Build history of the part. All positions in model axes, mm. A direction names the side the tool comes from. Give positions to 0.01 mm unless a question says otherwise; leave off trailing zeros. Loops run counter-clockwise (first coordinate to the right, second up) from the corner with the lowest first, then second, coordinate; pieces in that order, holes last. Notation, with made-up numbers: M 8,83.5 L 22,83.5 A24 ccw 22,100.5 Z; hole C 80.25,33 d2. An arc over 180 degrees is marked long. Put each result on its own line as item: value.
```python
from build123d import *

# Parameters (mm, degrees)
SKETCH_1_W               = 40
SKETCH_1_H               = 40
EXTRUDE_1_DEPTH          = 12.7
CUT_EXTRUDE_2_DEPTH      = 0.7
CUT_EXTRUDE_2_DEPTH_BACK = 1.5
SKETCH_8_W               = 36.4
SKETCH_8_H               = 28.4
CUT_EXTRUDE_4_DEPTH      = 12.7
SKETCH_10_R              = 0.5
SKETCH_10_R_2            = 1.5
SKETCH_10_W              = 3
SKETCH_10_H              = 13
EXTRUDE_2_DEPTH          = 2.2
CUT_EXTRUDE_START        = -12.7
SKETCH_13_R              = 1.35
CUT_EXTRUDE_6_DEPTH      = 12.7
FILLET_1_R               = 1
SKETCH_14_W              = 8.31999735
SKETCH_14_H              = 2.64999918
CUT_EXTRUDE_8_DEPTH      = 5.8
SKETCH_15_W              = 12.8999835
SKETCH_15_H              = 7.3
CUT_EXTRUDE_9_DEPTH      = 5.8
SKETCH_16_W              = 1.085536683
SKETCH_16_H              = 5.100270408
CUT_EXTRUDE_10_DEPTH     = 1.8
SKETCH_17_W              = 8.31999735
SKETCH_17_H              = 2.65925193
CUT_EXTRUDE_11_DEPTH     = 5.8
SKETCH_23_W              = 6.0022214
SKETCH_23_H              = 5.598076211
SKETCH_23_H_2            = 5.598076212
CUT_EXTRUDE_12_DEPTH     = 4
SKETCH_24_W              = 11
SKETCH_24_H              = 14
CUT_EXTRUDE_14_DEPTH     = 1.4


with BuildPart() as part:
    # 草图1 → 凸台-拉伸1 (new body)
    with BuildSketch(Plane(origin=(0, 0, -12.4), x_dir=(-1, 0, 0), z_dir=(0, 0, -1))):
        with Locations((-18.22949197, 11.132690632)):
            Rectangle(SKETCH_1_W, SKETCH_1_H)
    extrude(amount=-EXTRUDE_1_DEPTH)

    # 草图2 → 切除-拉伸2 (cut, two sides: drawn at the far end of the back side and taken through both)
    with BuildSketch(Plane.XY.offset(-8).offset(-CUT_EXTRUDE_2_DEPTH_BACK)):
        Polygon((-2.01828663, -8.469233156), (2.73171337, -8.469233156), (4.23171337, -5.871156945), (2.72949197, -3.269233156), (-2.01828663, -3.269233156), align=None)
        Polygon((-2.01828663, 25.534614421), (-2.01828663, 30.734614421), (2.73171337, 30.734614421), (4.23171337, 28.13653821), (2.72949197, 25.534614421), align=None)
        Polygon((38.47727057, 30.734614421), (33.72727057, 30.734614421), (32.22727057, 28.13653821), (33.72949197, 25.534614421), (38.47727057, 25.534614421), align=None)
        Polygon((38.47727057, -3.269233156), (38.47727057, -8.469233156), (33.72727057, -8.469233156), (32.22727057, -5.871156945), (33.72949197, -3.269233156), align=None)
    extrude(amount=CUT_EXTRUDE_2_DEPTH + CUT_EXTRUDE_2_DEPTH_BACK, mode=Mode.SUBTRACT)

    # 草图8 → 切除-拉伸4 (cut)
    with BuildSketch(Plane(origin=(0, 0, -12.4), x_dir=(-1, 0, 0), z_dir=(0, 0, -1))):
        with Locations((-18.22949197, 11.132690632)):
            Rectangle(SKETCH_8_W, SKETCH_8_H)
    extrude(amount=-CUT_EXTRUDE_4_DEPTH, mode=Mode.SUBTRACT)

    # 草图13 → 切除-拉伸6 (cut)
    with BuildSketch(Plane(origin=(0, 0, -12.4), x_dir=(-1, 0, 0), z_dir=(0, 0, -1)).offset(CUT_EXTRUDE_START)):
        with Locations((-35.22949197, -5.867309368)):
            Circle(SKETCH_13_R)
        with Locations(Location((-1.22949197, -5.867309368, 0), (0, 0, 180))):
            Circle(SKETCH_13_R)
        with Locations((-1.22949197, 28.132690632)):
            Circle(SKETCH_13_R)
        with Locations(Location((-35.22949197, 28.132690632, 0), (0, 0, 180))):
            Circle(SKETCH_13_R)
    extrude(amount=CUT_EXTRUDE_6_DEPTH, mode=Mode.SUBTRACT)

    # 圆角1
    fillet_1_edges = [part.edges().sort_by_distance(p)[0] for p in [
        (0.02949197, 25.332690632, -6.05),
        (0.02949197, -3.067309368, -6.05),
        (36.42949197, -3.067309368, -6.05),
        (36.42949197, 25.332690632, -6.05),
    ]]
    fillet(fillet_1_edges, radius=FILLET_1_R)

    # 草图14 → 切除-拉伸8 (cut)
    with BuildSketch(Plane.XZ.offset(8.867309368)):
        with Locations((8.169941285, -11.07500041)):
            Rectangle(SKETCH_14_W, SKETCH_14_H)
    extrude(amount=-CUT_EXTRUDE_8_DEPTH, mode=Mode.SUBTRACT)

    # 草图15 → 切除-拉伸9 (cut)
    with BuildSketch(Plane.XZ.offset(8.867309368)):
        with Locations((23.79587104, -8.75)):
            Rectangle(SKETCH_15_W, SKETCH_15_H)
    extrude(amount=-CUT_EXTRUDE_9_DEPTH, mode=Mode.SUBTRACT)

    # 草图16 → 切除-拉伸10 (cut)
    with BuildSketch(Plane(origin=(38.22949197, 0, 0), x_dir=(0, 0, -1), z_dir=(1, 0, 0))):
        with Locations((11.857231659, 0.566559812)):
            Rectangle(SKETCH_16_W, SKETCH_16_H)
    extrude(amount=-CUT_EXTRUDE_10_DEPTH, mode=Mode.SUBTRACT)

    # 草图17 → 切除-拉伸11 (cut)
    with BuildSketch(Plane(origin=(0, 31.132690632, 0), x_dir=(1, 0, 0), z_dir=(0, 1, 0))):
        with Locations((28.372981895, 11.070374035)):
            Rectangle(SKETCH_17_W, SKETCH_17_H)
    extrude(amount=-CUT_EXTRUDE_11_DEPTH, mode=Mode.SUBTRACT)

    # 草图23 → 切除-拉伸12 (cut)
    with BuildSketch(Plane.XY.offset(2.5)):
        with Locations((35.22838127, 28.333652527)):
            Rectangle(SKETCH_23_W, SKETCH_23_H)
        with Locations((35.22838127, -6.068271262)):
            Rectangle(SKETCH_23_W, SKETCH_23_H_2)
        with Locations((1.23060267, -6.068271262)):
            Rectangle(SKETCH_23_W, SKETCH_23_H_2)
        with Locations((1.23060267, 28.333652527)):
            Rectangle(SKETCH_23_W, SKETCH_23_H)
    extrude(amount=-CUT_EXTRUDE_12_DEPTH, mode=Mode.SUBTRACT)


with BuildPart() as body_2:
    # 草图10 → 凸台-拉伸2 (new body)
    with BuildSketch(Plane.XY.offset(0.3)):
        Polygon((-1.77050803, 25.534614421), (4.23171337, 25.534614421), (4.23171337, 31.132690632), (32.22727057, 31.132690632), (32.22727057, 25.534614421), (38.22949197, 25.534614421), (38.22949197, -3.269233156), (32.22727057, -3.269233156), (32.22727057, -8.867309368), (4.23171337, -8.867309368), (4.23171337, -3.269233156), (-1.77050803, -3.269233156), align=None)
        with Locations((18.22949197, 11.132690632)):
            Circle(SKETCH_10_R, mode=Mode.SUBTRACT)
        with Locations((3.22949197, 0.632690632)):
            Circle(SKETCH_10_R_2, mode=Mode.SUBTRACT)
        with Locations((3.22949197, 21.632690632)):
            Circle(SKETCH_10_R_2, mode=Mode.SUBTRACT)
        with Locations(Location((33.22949197, 21.632690632, 0), (0, 0, 180))):
            Circle(SKETCH_10_R_2, mode=Mode.SUBTRACT)
        with Locations(Location((33.22949197, 0.632690632, 0), (0, 0, 180))):
            Circle(SKETCH_10_R_2, mode=Mode.SUBTRACT)
        with Locations((3.22949197, 11.132690632)):
            Rectangle(SKETCH_10_W, SKETCH_10_H, mode=Mode.SUBTRACT)
        with Locations((33.22949197, 11.132690632)):
            Rectangle(SKETCH_10_W, SKETCH_10_H, mode=Mode.SUBTRACT)
    extrude(amount=EXTRUDE_2_DEPTH)

    # 草图24 → 切除-拉伸14 (cut)
    with BuildSketch(Plane(origin=(0, 0, 0.3), x_dir=(-1, 0, 0), z_dir=(0, 0, -1))):
        with Locations((-18.22949197, 11.132690632)):
            Rectangle(SKETCH_24_W, SKETCH_24_H)
    extrude(amount=-CUT_EXTRUDE_14_DEPTH, mode=Mode.SUBTRACT)

    # 草图22 → 切除-旋转3 (revolve, cut)
    with BuildSketch(Plane(origin=(0, 11.132690632, 0), x_dir=(-1, 0, 0), z_dir=(0, -1, 0))):
        Polygon((-18.72949197, -1.7), (-19.400771675, -2.5), (-18.22949197, -2.5), (-18.22949197, -1.7), align=None)
    revolve(axis=Axis((18.22949197, 11.132690632, 5.06186702), (0, 0, -1)), mode=Mode.SUBTRACT)

    # Combine 1: union part
    add(part.part)


solid = body_2.part
```
Q1. Slice it at B-B (y = 14). List the corners of the cut face in (x, z), and give its area (3 significant figures).
Here are the results:
outline: M -1.77,-12.4 L 0.03,-12.4 L 0.03,0.3 L 1.73,0.3 L 1.73,2.5 L -1.77,2.5 Z; M 4.73,0.3 L 12.73,0.3 L 12.73,1.7 L 23.73,1.7 L 23.73,0.3 L 31.73,0.3 L 31.73,2.5 L 4.73,2.5 Z; M 34.73,0.3 L 36.43,0.3 L 36.43,-12.4 L 38.23,-12.4 L 38.23,2.5 L 34.73,2.5 Z
area: 105 mm²
Q2. Slice it at A-A (z = -0.75). List the corners of the cut face in (x, y), and give its area (3 significant figures).
Here are the results:
outline: M -1.77,-3.27 L 4.23,-3.27 L 4.23,-8.87 L 32.23,-8.87 L 32.23,-3.27 L 38.23,-3.27 L 38.23,25.53 L 32.23,25.53 L 32.23,31.13 L 4.23,31.13 L 4.23,25.53 L -1.77,25.53 Z; hole M 0.03,-2.07 A1 ccw 1.03,-3.07 L 35.43,-3.07 A1 ccw 36.43,-2.07 L 36.43,24.33 A1 ccw 35.43,25.33 L 1.03,25.33 A1 ccw 0.03,24.33 Z
area: 433 mm²
Q3. Slice it at D-D (z = -10.25). List the corners of the cut face in (x, y).
Here are the results:
outline: M -1.77,-8.87 L 4.01,-8.87 L 4.01,-3.07 L 1.03,-3.07 A1 cw 0.03,-2.07 L 0.03,24.33 A1 cw 1.03,25.33 L 24.21,25.33 L 24.21,31.13 L -1.77,31.13 Z; M 12.33,-8.87 L 17.35,-8.87 L 17.35,-3.07 L 12.33,-3.07 Z; M 30.25,-8.87 L 38.23,-8.87 L 38.23,31.13 L 32.53,31.13 L 32.53,25.33 L 35.43,25.33 A1 cw 36.43,24.33 L 36.43,-2.07 A1 cw 35.43,-3.07 L 30.25,-3.07 Z; hole C 1.23,-5.87 d2.7; hole C 1.23,28.13 d2.7; hole C 35.23,-5.87 d2.7; hole C 35.23,28.13 d2.7
Q4. Slice it at C-C (x = 11.5). List the corners of the cut face in (y, z).
Here are the results:
outline: M -8.87,-9.75 L -3.07,-9.75 L -3.07,0.3 L 25.33,0.3 L 25.33,-12.4 L 31.13,-12.4 L 31.13,2.5 L -8.87,2.5 Z
Q5. Probe line 1 (X direction, y = 6, z = 1.25); line 2 (Y direction, x = 9, z = 0); line 3 (X direction, y = -1.5, z = -9). List the from-to ranges inside material, lowest first. Write a range as from..to.
Here are the results:
line 1: -1.77..1.73, 4.73..12.73, 23.73..31.73, 34.73..38.23
line 2: -8.87..-3.07, 25.33..31.13
line 3: -1.77..0.03, 36.43..38.23
Q6. Drop flat-ended pins along their axis: pin 1 Ø2.5 at (x, z) = (34, 1.5) entering from +Y; pin 2 Ø1.6 at (x, y) = (1.23, -5.87) entering from +Z; pin 3 Ø5.5 at (x, y) = (16, 9) entering from -Z; pin 4 Ø3 at (y, z) = (-7.5, 0.5) entering from -X. Give the stop position or say it passes through.
Here are the results:
pin 1: y = 25.53
pin 2: through
pin 3: z = 1.7
pin 4: x = 4.23
Q7. Mould opens along X. For faces 1 (the flat face through (35, 30, -1.5)), 2 (the flat face through (32.988, 29.454, -8.415)), 3 (the flat face through (3.49, 26.85, -8.42)), 4 (the cylindrical face through (36.58, -5.81, -10.93)) say: pulls with the +X half, pulls with the -X half, needs draft (parallel to the pull), parting line crosses it, or undercut.
Here are the results:
face 1: needs draft
face 2: pulls with the +X half
face 3: pulls with the -X half
face 4: undercut
Q8. Tool access for faces 5 (the flat face through (37, -1.984, -12)), 6 (the flat face through (8, -6, -9.75)), 7 (the flat face through (0, 29, -7.3)): list every direction of +Z, -Z, +X, -X, +Y, -Y with a clear straight run to the whole face (end or side of a thin tool).
Here are the results:
face 5: -Z, +X
face 6: -Z, -Y
face 7: -X
